from build123d import *

# Parameters (mm, degrees)
SKETCH1_R           = 16.1
BOSS_EXTRUDE1_DEPTH = 0.01
FILLET1_R           = 5
SKETCH2_R           = 12
BOSS_EXTRUDE2_DEPTH = 17
CHAMFER1_SIZE       = 17
CHAMFER1_SIZE_2     = 11.90352815


with BuildPart() as part:
    # Sketch1 → Boss-Extrude1 (new body)
    with BuildSketch(Plane(origin=(0, 0, 0), x_dir=(0, 0, -1), z_dir=(1, 0, 0))):
        with Locations(Location((0, 0, 0), (0, 0, 180))):
            Circle(SKETCH1_R)
    extrude(amount=BOSS_EXTRUDE1_DEPTH)

    # Fillet1
    # the kernel refuses this fillet: 5 mm, written as the material it takes off along each edge
    with BuildSketch(Plane(origin=(0.01, 0, 0), x_dir=(0, 0, 1), z_dir=(0, 1, 0))) as fillet1_piece_1:
        with BuildLine():
            CenterArc((15.783930387, -5), FILLET1_R, 86.375692506, 3.624307494)
            Line((15.783930387, 0), (16.1, 0))
            Line((16.1, 0), (16.1, -0.01))
        make_face()
    revolve(axis=Axis((0.01, 0, 0), (1, 0, 0)), mode=Mode.SUBTRACT)

    # Sketch2 → Boss-Extrude2 (add)
    with BuildSketch(Plane(origin=(0.01, 0, 0), x_dir=(0, 0, -1), z_dir=(1, 0, 0))):
        Circle(SKETCH2_R)
    extrude(amount=BOSS_EXTRUDE2_DEPTH)

    # Chamfer1
    # the kernel refuses this chamfer: 17, 11.90352815 mm, written as the material it takes off along each edge
    with BuildSketch(Plane(origin=(17.01, 0, 0), x_dir=(0, 0, -1), z_dir=(0, -1, 0))) as chamfer1_piece_1:
        Polygon((12, -CHAMFER1_SIZE), (12 - CHAMFER1_SIZE_2, 0), (12, 0), align=None)
    revolve(axis=Axis((17.01, 0, 0), (1, 0, 0)), mode=Mode.SUBTRACT)


solid = part.part
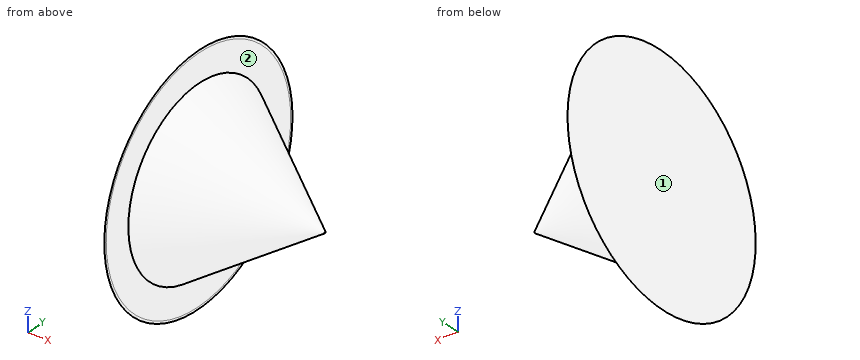
CAD build for the part. Positions are in the model's coordinates, mm. Face numbers are marked on the shaded views. A direction names the side the tool comes from. Round coordinates to 2 decimals unless told otherwise and drop trailing zeros. Write each loop counter-clockwise with the first axis right and the second up, starting at its lowest first coordinate (ties: lowest second). Pieces come first, ordered by that corner, then holes. Notation, with made-up numbers: M -6.75,46.25 L 43.25,46.25 A25 cw 43.25,70.25 Z; hole C -31,3 d2. An arc over 180 degrees is marked long. Use a Markdown table: item, result. Add a question column.
1. Flat gauge pins, fed straight in: P1, Ø5, axis at x = 12.5, y = -0.5, coming from the +Z side; P2, Ø4, axis at y = 7.5, z = 6, coming from the +X side. Where does each tip first touch, or does it go through?
2. Drill centre lines: probe 1 along X at (y, z) = (6, -5); probe 2 along Y at (x, z) = (9.25, -1); probe 3 along X at (y, z) = (-7.5, -7.5). Where is each one in solid material? Low to high.
3. 3-axis set-ups, long thin cutter, end or side, ignore diameter. For the marked faces 1 and 2: which of +Z, -Z, +X, -X, +Y, -Y reach the whole face in a straight line?
4. Slice it at B-B on x = 1.5. Give the cut face in (y, z), then the cut area to 3 significant figures.
5. Slice it at A-A on x = 9.25. Give the cut face in (y, z).
Reply:
| question | item | result |
|---|---|---|
| 1 | P1 | stops at z = 4.99 |
| 1 | P2 | stops at x = 6.29 |
| 2 | probe 1 | x = 0 to 5.99 |
| 2 | probe 2 | y = -5.44 to 5.44 |
| 2 | probe 3 | x = 0 to 2 |
| 3 | face 1 | +Z, -Z, -X, +Y, -Y |
| 3 | face 2 | +X |
| 4 | outline | C 0,0 d21.91 |
| 4 | area | 377 mm^2 |
| 5 | outline | C 0,0 d11.06 |
